from build123d import *

# Parameters (mm, degrees)
HOLE_WIZARD_M16_1_D     = 14
HOLE_WIZARD_M16_1_DEPTH = 38
HOLE_WIZARD_M16_1_TIP   = 4.206024333
CHAMFER_1_SIZE          = 10
FILLET_1_R              = 10


with BuildPart() as part:
    # 草图1 → 旋转1 (revolve)
    with BuildSketch(Plane.XY, mode=Mode.PRIVATE) as revolve_1_sk:
        Polygon((0, 0), (85, 0), (85, -25), (117.5, -25), (117.5, -150), (67.5, -150), (67.5, -110), (0, -110), align=None)
    revolve(revolve_1_sk.sketch.rotate(Axis((0, 0, 0), (0, 1, 0)), 90), axis=Axis((0, 0, 0), (0, 1, 0)))

    # M16 螺纹孔1
    with Locations(Plane(origin=(0, -110, 0), x_dir=(-1, 0, 0), z_dir=(0, -1, 0))):
        with Locations((0, 0)):
            Hole(HOLE_WIZARD_M16_1_D / 2, depth=HOLE_WIZARD_M16_1_DEPTH)
            with Locations((0, 0, -(HOLE_WIZARD_M16_1_DEPTH + HOLE_WIZARD_M16_1_TIP / 2))):  # 118° drill point
                Cone(0, HOLE_WIZARD_M16_1_D / 2, HOLE_WIZARD_M16_1_TIP, mode=Mode.SUBTRACT)

    # 倒角1
    chamfer_1_edges = [part.edges().sort_by_distance(p)[0] for p in [
        (0, -150, 117.5),
    ]]
    chamfer(chamfer_1_edges, length=CHAMFER_1_SIZE)

    # 圆角1
    fillet_1_edges = [part.edges().sort_by_distance(p)[0] for p in [
        (0, -25, 117.5),
    ]]
    fillet(fillet_1_edges, radius=FILLET_1_R)


solid = part.part
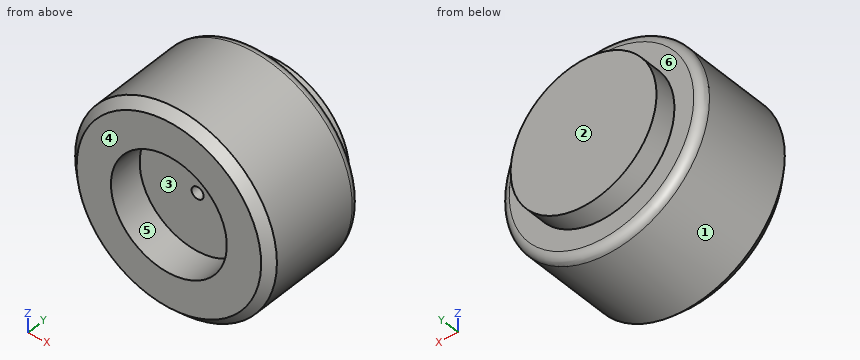
Source: CAD feature listing. Evaluate the final solid. Frame: model axes, mm. Face numbers are marked on the shaded views. A direction names the side the tool comes from. Round coordinates to 2 decimals unless told otherwise and drop trailing zeros. Order: outer loops, then holes, each group sorted by start corner. A loop starts at its lowest first (then second) coordinate and runs counter-clockwise, first axis right, second up. Notation, with made-up numbers: (59.5, -6.75) - (70.5, -6.75) arc R16 ccw to (70.5, 23.25) - close; hole circle Ø9 at (25, 67.25). An arc over 180 degrees is marked (long way). Use a Markdown table: item, result. Add a question column.
1. First-contact query: pin 1 (3 mm diameter, centred on y = -40.5, z = 81.5, fed in from +X); pin 2 (6 mm diameter, centred on y = -116, z = -35.5, fed in from -X); pin 3 (1.5 mm diameter, centred on y = -75, z = -91.5, fed in from -X); pin 4 (16 mm diameter, centred on x = 0, z = 0, fed in from +Y). Flat tips, straight axial feed; report the tip coordinate or a pass-through.
2. Mould query, pull axis Z, two halves, no side actions, for the marked faces 1, 2 and 3. Classes: +Z half, -Z half, draft (parallel to the pull), parting line (faces both ways), or undercut.
3. Line query: probe 1 along X at (y, z) = (-136, 0); probe 2 along Y at (x, z) = (42, 36); probe 3 along Z at (x, y) = (-3, -98.5). Output: solid intervals per line, ascending.
4. Section query B-B (y = -12). Return the cut outline in (x, z).
5. Set-up query: the marked faces 4, 5 and 6. Return all of +Z, -Z, +X, -X, +Y, -Y with unobstructed straight access to the full face (end or side cutting, diameter ignored); none if empty.
6. Section query A-A (y = -136). Return the cut outline in (x, z).
Derived:
| question | item | result |
|---|---|---|
| 1 | pin 1 | x = 86.06 |
| 1 | pin 2 | x = -112.92 |
| 1 | pin 3 | x = -74.64 |
| 1 | pin 4 | y = 0 |
| 2 | face 1 | parting line |
| 2 | face 2 | draft |
| 2 | face 3 | undercut |
| 3 | probe 1 | -117.5 to -67.5, 67.5 to 117.5 |
| 3 | probe 2 | -110 to 0 |
| 3 | probe 3 | -117.46 to -6.32, 6.32 to 117.46 |
| 4 | outline | circle Ø170 at (0, 0) |
| 5 | face 4 | +Z, -Z, +X, -X, -Y |
| 5 | face 5 | -Y |
| 5 | face 6 | +Y |
| 6 | outline | circle Ø235 at (0, 0); hole circle Ø135 at (0, 0) |
